Could you check a few things on this model? Use its own coordinates, in mm. Face numbers are marked on the shaded views. Coordinates: 2 decimals unless noted, no trailing zeros. Loops run counter-clockwise (first coordinate to the right, second up) from the corner with the lowest first, then second, coordinate; pieces in that order, holes last.
Autodesk Inventor part; units mm, degrees
ref_plane "YZ Plane" through (0, 0, 0) normal (1, 0, 0) x (0, 1, 0)
ref_plane "XZ Plane" through (0, 0, 0) normal (0, 1, 0) x (-1, 0, 0)
ref_plane "XY Plane" through (0, 0, 0) normal (0, 0, 1) x (1, 0, 0)
sketch "Sketch1" plane through (0, 0, 0) normal (0, 0, 1) x (1, 0, 0)
  circle A0 centre (0, 0) radius 91.2813
  dimension "d0" = 182.5625
extrude "Extrusion1" add sketch "Sketch1" along normal blind 25.4
fillet "Fillet1" radius 19.05 1 edges at (-91.2813, 0, 25.4)
shell "Shell1" thickness 17.78 removed faces 1 at (21.5393, 24.1816, 0)
properties part number "speakerGrill"
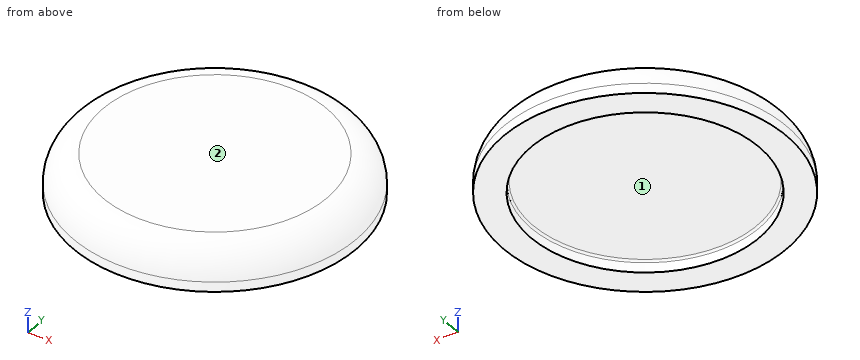
(1) I need wall thicknesses on probe 1 along Y at (x, z) = (0, 3.25); probe 2 along Z at (x, y) = (-46, -56); probe 3 along Y at (x, z) = (47, 15.5). Which ranges of each line are inside material? Lowest first, please.
Answers:
probe 1: y = -91.28 to -73.5, 73.5 to 91.28
probe 2: z = 7.6 to 25.4
probe 3: y = -75.51 to 75.51
(2) Imagine slicing it at A-A, the plane x = 0. Write out the boundary of the cut face in (y, z).
Answers:
outline: (-91.28, 0) - (-73.5, 0) - (-73.5, 6.35) arc R1.27 cw to (-72.23, 7.62) - (72.23, 7.62) arc R1.27 cw to (73.5, 6.35) - (73.5, 0) - (91.28, 0) - (91.28, 6.35) arc R19.05 ccw to (72.23, 25.4) - (-72.23, 25.4) arc R19.05 ccw to (-91.28, 6.35) - close
(3) We'd pull the mould along Y, two halves only. Please class the marked faces 1 and 2: +Y half, -Y half, draft (parallel to the pull), parting line (faces both ways), or undercut.
Answers:
face 1: undercut
face 2: draft
(4) Imagine slicing it at C-C, the plane z = 2.5. Write out the boundary of the cut face in (x, y).
Answers:
outline: circle Ø182.56 at (0, 0); hole circle Ø147 at (0, 0)
(5) For pin 1 (8 mm diameter, centred on x = 17, z = 16, fed in from +Y); pin 2 (2 mm diameter, centred on y = 39.5, z = 14.5, fed in from +X); pin 3 (10 mm diameter, centred on y = 23.5, z = 7.5, fed in from +X), each with a flat end and sliding along its axis, tell me the tip position at first contact or that it passes through.
Answers:
pin 1: stops at y = 89
pin 2: stops at x = 80.95
pin 3: stops at x = 89.37
